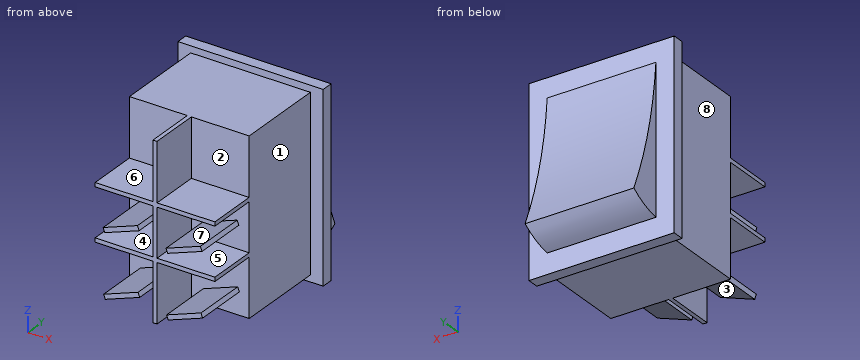
```python
from build123d import *

# Parameters (mm, degrees)
EXTRUDE1_DEPTH     = 14.85
SKETCH2_W          = 25
SKETCH2_H          = 2
EXTRUDE2_DEPTH     = 1.15
EXTRUDE4_DEPTH     = 9.35
SKETCH5_W          = 9.95
SKETCH5_H          = 10
SKETCH5_H_2        = 8.3
CUT_EXTRUDE1_DEPTH = 8.7
EXTRUDE5_DEPTH     = 9.3


with BuildPart() as part:
    # Sketch1 → Extrude1 (new body, symmetric)
    with BuildSketch(Plane.XY):
        Polygon((12.5, 26.2), (-12.5, 26.2), (-12.5, 24.2), (-10.3, 24.2), (-10.3, 0), (10.3, 0), (10.3, 24.2), (12.5, 24.2), align=None)
    extrude(amount=EXTRUDE1_DEPTH, both=True)

    # Sketch2 → Extrude2 (add)
    with BuildSketch(Plane.XY.offset(14.85)):
        with Locations((0, 25.2)):
            Rectangle(SKETCH2_W, SKETCH2_H)
    extrude2 = extrude(amount=EXTRUDE2_DEPTH)

    # Mirror1: Extrude2 across plane
    add(extrude2.mirror(Plane.XY))

    # Sketch4 → Extrude4 (add, symmetric)
    with BuildSketch(Plane(origin=(0, 0, 0), x_dir=(0, 0, -1), z_dir=(1, 0, 0))):
        with BuildLine():
            Line((-12.7, 26.2), (-12.7, 26.21))
            ThreePointArc((-12.7, 26.21), (-0.971928332, 28.066601365), (10.3, 31.8))
            ThreePointArc((10.3, 31.8), (11.738824473, 29.133109614), (12.5, 26.2))
            Line((12.5, 26.2), (-12.7, 26.2))
        make_face()
    extrude(amount=EXTRUDE4_DEPTH, both=True)

    # Sketch5 → Cut-Extrude1 (cut)
    with BuildSketch(Plane.XZ):
        with Locations((5.325, 9.85)):
            Rectangle(SKETCH5_W, SKETCH5_H)
        with Locations((5.325, 0)):
            Rectangle(SKETCH5_W, SKETCH5_H_2)
        with Locations((-5.325, 9.85)):
            Rectangle(SKETCH5_W, SKETCH5_H)
        with Locations((-5.325, -9.85)):
            Rectangle(SKETCH5_W, SKETCH5_H)
        with Locations((5.325, -9.85)):
            Rectangle(SKETCH5_W, SKETCH5_H)
        with Locations((-5.325, 0)):
            Rectangle(SKETCH5_W, SKETCH5_H_2)
    extrude(amount=-CUT_EXTRUDE1_DEPTH, mode=Mode.SUBTRACT)

    # Sketch9 → Extrude5 (add)
    with BuildSketch(Plane.XZ.offset(-8.7)):
        Polygon((-8.145589208, -13.205654355), (-2.225525697, -11.050927452), (-2.499141811, -10.299173355), (-8.419205322, -12.453900258), align=None)
        Polygon((2.678569935, -13.205654355), (8.598633446, -11.050927452), (8.325017331, -10.299173355), (2.40495382, -12.453900258), align=None)
        Polygon((-8.241705742, -2.392544248), (-2.321642231, -0.237817345), (-2.595258346, 0.513936752), (-8.515321856, -1.640790151), align=None)
        Polygon((2.582453401, -2.392544248), (8.502516912, -0.237817345), (8.228900797, 0.513936752), (2.308837286, -1.640790151), align=None)
    extrude(amount=EXTRUDE5_DEPTH)


solid = part.part
```
Read the model definition and answer for the solid it produces. Units are mm, in the model's axes. Face numbers are marked on the shaded views. A direction names the side the tool comes from. Give positions to 0.01 mm unless a question says otherwise; leave off trailing zeros. Loops run counter-clockwise (first coordinate to the right, second up) from the corner with the lowest first, then second, coordinate; pieces in that order, holes last.
Item 1: For the marked faces 1, 2, 3, 4 and 5, determine the directions among +Z, -Z, +X, -X, +Y, -Y from which every point of the face is accessible in a straight line to the end or side of a thin tool.
Item 2: Each of these flat-tipped pins is pushed along its axis until it touches: pin 1 Ø7 at (x, y) = (7, 5) entering from -Z; pin 2 Ø9.5 at (x, y) = (-7.5, 5.5) entering from +Z; pin 3 Ø1 at (y, z) = (4, 10) entering from +X; pin 4 Ø5 at (x, z) = (-2, 1) entering from -Y. Where does it stop, or does it pass through?
Item 3: The part is cut by section B-B (z = 7). Write down the section's boundary in (x, y).
Item 4: The mould has two halves that part along X. Classify the marked faces 6, 7 and 8: released by +X, released by -X, zero draft, split by the parting line, or undercut.
Item 5: The part is cut by section D-D (z = -5.5). Write down the section's boundary in (x, y).
Item 6: Find the intervals of material crossed by line 1 along Z through (x, y) = (-5, 5.5); line 2 along Z through (x, y) = (9, 6.5); line 3 along Z through (x, y) = (0.75, 12.5), in increasing order.
Item 7: The part is cut by section C-C (y = 20.5). Write down the section's boundary in (x, z).
Taken from the geometry:
1. face 1: +Z, -Z, +X, -Y
1. face 2: +Z, +X, -Y
1. face 3: -Z, -Y
1. face 4: -X, -Y
1. face 5: +X, -Y
2. pin 1: stops at z = -12.91
2. pin 2: stops at z = 14.85
2. pin 3: stops at x = 0.35
2. pin 4: stops at y = -0.6
3. outline: (-12.5, 24.2) - (-10.3, 24.2) - (-10.3, 8.7) - (-0.35, 8.7) - (-0.35, 0) - (0.35, 0) - (0.35, 8.7) - (10.3, 8.7) - (10.3, 24.2) - (12.5, 24.2) - (12.5, 26.2) - (9.35, 26.2) - (9.35, 26.87) - (-9.35, 26.87) - (-9.35, 26.2) - (-12.5, 26.2) - close
4. face 6: zero draft
4. face 7: undercut
4. face 8: released by -X
5. outline: (-12.5, 24.2) - (-10.3, 24.2) - (-10.3, 8.7) - (-0.35, 8.7) - (-0.35, 0) - (0.35, 0) - (0.35, 8.7) - (10.3, 8.7) - (10.3, 24.2) - (12.5, 24.2) - (12.5, 26.2) - (9.35, 26.2) - (9.35, 29.96) - (-9.35, 29.96) - (-9.35, 26.2) - (-12.5, 26.2) - close
6. line 1: z = -12.06 to -11.21, -4.85 to -4.15, -1.21 to -0.36, 4.15 to 4.85
6. line 2: z = -4.85 to -4.15, 4.15 to 4.85
6. line 3: z = -14.85 to 14.85
7. outline: (-10.3, -14.85) - (10.3, -14.85) - (10.3, 14.85) - (-10.3, 14.85) - close
